Verification items for the finished model (mm, model axes). Coordinates: 2 decimals unless noted, no trailing zeros. Write each loop counter-clockwise with the first axis right and the second up, starting at its lowest first coordinate (ties: lowest second). Pieces come first, ordered by that corner, then holes.
```python
from build123d import *

# Parameters (mm, degrees)
F1_DEPTH = 5
F2_R     = 2.655635
F3_R     = 2.656


with BuildPart() as f1:
    # F0 (on Top) → F1 (new body)
    with BuildSketch(Plane.XY):
        with BuildLine():
            Line((-82.867503, -15.946694), (82.867503, -15.946694))
            Line((82.867503, -15.946694), (82.867503, -4.053306))
            ThreePointArc((82.867503, -4.053306), (77.009639, 10.088829), (62.867503, 15.946694))
            Line((62.867503, 15.946694), (-62.867503, 15.946694))
            ThreePointArc((-62.867503, 15.946694), (-77.009639, 10.088829), (-82.867503, -4.053306))
            Line((-82.867503, -4.053306), (-82.867503, -15.946694))
        make_face()
    extrude(amount=F1_DEPTH)

    # F2
    f2_edges = [f1.edges().sort_by_distance(p)[0] for p in [
        (-82.867503, -15.946694, 2.5),
    ]]
    fillet(f2_edges, radius=F2_R)

    # F3
    f3_edges = [f1.edges().sort_by_distance(p)[0] for p in [
        (82.867503, -15.946694, 2.5),
    ]]
    fillet(f3_edges, radius=F3_R)


solid = f1.part
```
1. Sectioned sample at B-B, the plane y = 14.5. Record the boundary of the cut face in (x, z).
2. Sectioned sample at C-C, the plane y = 8.5. Record the boundary of the cut face in (x, z).
3. Material ranges on L1, parallel to X at y = 9, z = 3.15; L2, parallel to X at y = 8, z = 0.6; L3, parallel to Y at x = 70.5, z = 0.8, recorded low to high.
4. Sectioned sample at A-A, the plane z = 2.7. Record the boundary of the cut face in (x, y), and give its area (3 significant figures).
5. Gauge pin test, flat ends, axial feed: P1, Ø1, axis at y = 10, z = 3.5, coming from the +X side; P2, Ø1.5, axis at y = 6.5, z = 4, coming from the +X side; P3, Ø1.5, axis at y = 5, z = 4.5, coming from the +X side. Record the tip position at first contact, or that the pin passes through.
Outcome:
1. outline: (-70.34, 0) - (70.34, 0) - (70.34, 5) - (-70.34, 5) - close
2. outline: (-78.44, 0) - (78.44, 0) - (78.44, 5) - (-78.44, 5) - close
3. L1: x = -78.02 to 78.02
3. L2: x = -78.83 to 78.83
3. L3: y = -15.95 to 14.43
4. outline: (-82.87, -13.29) arc R2.66 ccw to (-80.21, -15.95) - (80.21, -15.95) arc R2.66 ccw to (82.87, -13.29) - (82.87, -4.05) arc R20 ccw to (62.87, 15.95) - (-62.87, 15.95) arc R20 ccw to (-82.87, -4.05) - close
4. area: 5,110 mm2
5. P1: stops at x = 77.57
5. P2: stops at x = 80.3
5. P3: stops at x = 81.06
